```python
from build123d import *

# Parameters (mm, degrees)
BOSS_EXTRUDE2_DEPTH = 12.7
SKETCH2_W           = 12.7
SKETCH2_H           = 6.35
BOSS_EXTRUDE3_DEPTH = 38.1
SKETCH3_W           = 6.35
SKETCH3_H           = 12.7
BOSS_EXTRUDE5_DEPTH = 6.096
BOSS_EXTRUDE5_DRAFT = -15
SKETCH4_W           = 12.7
SKETCH4_H           = 38.1
BOSS_EXTRUDE6_DEPTH = 2.54
SKETCH5_R           = 2.54
CUT_EXTRUDE1_DEPTH  = 8.89


with BuildPart() as part:
    # Sketch1 → Boss-Extrude2 (new body)
    with BuildSketch(Plane.XY):
        Polygon((12.7, 0), (19.05, 0), (19.05, 6.35), (12.7, 6.35), (12.7, 44.45), (0, 44.45), (0, 6.35), (-6.35, 6.35), (-6.35, 0), (0, 0), align=None)
    extrude(amount=BOSS_EXTRUDE2_DEPTH)

    # Sketch2 → Boss-Extrude3 (add)
    with BuildSketch(Plane(origin=(0, 44.45, 0), x_dir=(1, 0, 0), z_dir=(0, 1, 0))):
        with Locations((6.35, -3.175)):
            Rectangle(SKETCH2_W, SKETCH2_H)
    extrude(amount=BOSS_EXTRUDE3_DEPTH)


with BuildPart() as boss_extrude5_tool:
    # Sketch3 → Boss-Extrude5 (with draft: the straight prism first)
    with BuildSketch(Plane.XZ):
        with Locations((6.35, 6.35)):
            Rectangle(SKETCH3_W, SKETCH3_H)
    extrude(amount=BOSS_EXTRUDE5_DEPTH)
    # Boss-Extrude5: the draft: its side faces are tilted about the plane it starts from
    boss_extrude5_sides = [boss_extrude5_tool.faces().sort_by_distance(p)[0] for p in [
        (6.35, -3.048, 0),
        (9.525, -3.048, 6.35),
        (6.35, -3.048, 12.7),
        (3.175, -3.048, 6.35),
    ]]
    draft(boss_extrude5_sides, Plane.XZ, BOSS_EXTRUDE5_DRAFT)


with BuildPart() as part_1:
    add(part.part)

    # Boss-Extrude5: add boss_extrude5_tool
    add(boss_extrude5_tool.part)

    # Sketch4 → Boss-Extrude6 (add)
    with BuildSketch(Plane.XY.offset(6.35)):
        with Locations((6.35, 63.5)):
            Rectangle(SKETCH4_W, SKETCH4_H)
    extrude(amount=BOSS_EXTRUDE6_DEPTH)

    # Sketch5 → Cut-Extrude1 (cut)
    with BuildSketch(Plane.XY.offset(8.89)):
        with Locations((6.35, 76.2)):
            Circle(SKETCH5_R)
    extrude(amount=-CUT_EXTRUDE1_DEPTH, mode=Mode.SUBTRACT)


solid = part_1.part
```
The listing builds one solid part. Answer for the finished solid, in the listing's coordinates (mm). A direction names the side the tool comes from. Round coordinates to 2 decimals unless told otherwise and drop trailing zeros. Write each loop counter-clockwise with the first axis right and the second up, starting at its lowest first coordinate (ties: lowest second). Pieces come first, ordered by that corner, then holes. Notation, with made-up numbers: (19.25, -39) -> (57.25, -39) arc R20 cw to (57.25, -3) -> close; hole circle Ø1 at (21.25, 54.25). An arc over 180 degrees is marked (long way). Write item = value, one per line.
1) Given pin 1 (7.5 mm diameter, centred on x = 15.5, z = 9, fed in from -Y); pin 2 (10 mm diameter, centred on x = 8.5, y = 24, fed in from -Z); pin 3 (7 mm diameter, centred on x = -4, z = 7, fed in from +Y), each flat-ended and moving along its own axis, determine where each tip first touches the part or whether it passes through.
Check values:
pin_1 = 0
pin_2 = 0
pin_3 = 6.35
2) Section A-A on y = 76.2 is taken. Write down the section's boundary in (x, z).
Check values:
outline = (0, 0) -> (3.81, 0) -> (3.81, 8.89) -> (0, 8.89) -> close; (8.89, 0) -> (12.7, 0) -> (12.7, 8.89) -> (8.89, 8.89) -> close
3) Section B-B on z = 6.75 is taken. Write down the section's boundary in (x, y) (3 decimals), plus the area to 3 significant figures.
Check values:
outline = (-6.35, 0) -> (3.175, 0) -> (1.542, -6.096) -> (11.158, -6.096) -> (9.525, 0) -> (19.05, 0) -> (19.05, 6.35) -> (12.7, 6.35) -> (12.7, 82.55) -> (0, 82.55) -> (0, 6.35) -> (-6.35, 6.35) -> close; hole circle Ø5.08 at (6.35, 76.2)
area = 1,160 mm²
4) Which of the six approach directions +Z, -Z, +X, -X, +Y, -Y give full straight-line access (tool end or side, diameter ignored) to faces 5 (the flat face through (6, 44.45, 11)), 6 (the flat face through (14, 0, 6)), 7 (the flat face through (0, 44, 5)), 8 (the flat face through (2.37, -3.01, 6.24)), 9 (the flat face through (12.7, 44, 5))?
Check values:
face_5 = +Z, +X, -X, +Y
face_6 = +Z, -Z, +X
face_7 = +Z, -Z, -X, +Y
face_8 = +Z, -Z, -X
face_9 = +Z, -Z, +X, +Y
5) Section C-C on x = 6.35 is taken. Write down the section's boundary in (y, z), plus the area to 3 significant figures.
Check values:
outline = (-6.1, -1.63) -> (0, 0) -> (73.66, 0) -> (73.66, 8.89) -> (44.45, 8.89) -> (44.45, 12.7) -> (0, 12.7) -> (-6.1, 14.33) -> close; (78.74, 0) -> (82.55, 0) -> (82.55, 8.89) -> (78.74, 8.89) -> close
area = 945 mm²
6) For a pull along Y with two mould halves and no side action, classify faces 1 (the flat face through (6, -6.096, 6)), 2 (the flat face through (-6.35, 3, 6)), 3 (the flat face through (16, 6.35, 6)), 4 (the cylindrical face through (5.8, 73.72, 4.51)) as released by +Y, released by -Y, zero draft, split by the parting line, or undercut.
Check values:
face_1 = released by -Y
face_2 = zero draft
face_3 = released by +Y
face_4 = undercut
7) Straight lines are drawn through the part: line 1 along Y through (x, z) = (6.35, 3); line 2 along Y through (x, z) = (8.25, 12.5); line 3 along Y through (x, z) = (17, 0.75). For each, find the intervals that lie inside material, in ascending order. Write a range as [from, to].
Check values:
line_1 = [-6.1, 73.66], [78.74, 82.55]
line_2 = [-6.1, 44.45]
line_3 = [0, 6.35]
8) Section D-D on x = 15.75 is taken. Write down the section's boundary in (y, z).
Check values:
outline = (0, 0) -> (6.35, 0) -> (6.35, 12.7) -> (0, 12.7) -> close
